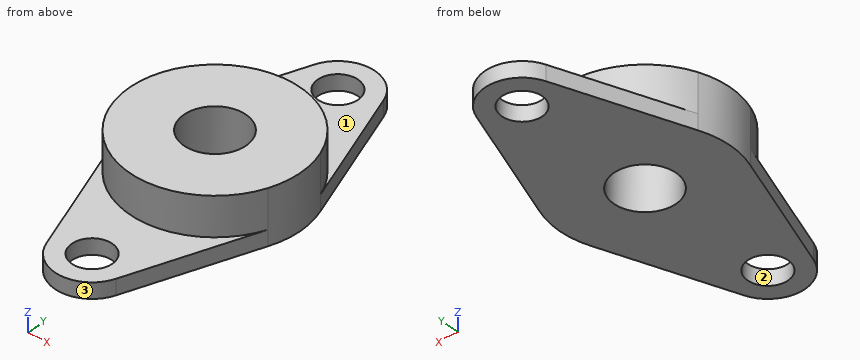
```python
from build123d import *

# Parameters (mm, degrees)
CROQUIS1_R              = 4
CROQUIS1_R_2            = 2.6
SALIENTE_EXTRUIR1_DEPTH = 7
CROQUIS2_R              = 2.6
CORTAR_EXTRUIR1_DEPTH   = 5


with BuildPart() as part:
    # Croquis1 → Saliente-Extruir1 (new body)
    with BuildSketch(Plane.XY):
        with BuildLine():
            Line((10.288824315, -3.891027397), (4.514634908, -19.880359362))
            ThreePointArc((4.514634908, -19.880359362), (0, -23.05), (-4.514634908, -19.880359362))
            Line((-4.514634908, -19.880359362), (-10.288824315, -3.891027397))
            ThreePointArc((-10.288824315, -3.891027397), (-11, 0), (-10.288824315, 3.891027397))
            Line((-10.288824315, 3.891027397), (-4.514634908, 19.880359362))
            ThreePointArc((-4.514634908, 19.880359362), (0, 23.05), (4.514634908, 19.880359362))
            Line((4.514634908, 19.880359362), (10.288824315, 3.891027397))
            ThreePointArc((10.288824315, 3.891027397), (11, 0), (10.288824315, -3.891027397))
        make_face()
        Circle(CROQUIS1_R, mode=Mode.SUBTRACT)
        with Locations((0, 18.25)):
            Circle(CROQUIS1_R_2, mode=Mode.SUBTRACT)
        with Locations((0, -18.25)):
            Circle(CROQUIS1_R_2, mode=Mode.SUBTRACT)
    extrude(amount=SALIENTE_EXTRUIR1_DEPTH)

    # Croquis2 → Cortar-Extruir1 (cut)
    with BuildSketch(Plane.XY.offset(7)):
        with BuildLine():
            Line((-4.514634908, 19.880359362), (-10.288824315, 3.891027397))
            ThreePointArc((-10.288824315, 3.891027397), (0, 11), (10.288824315, 3.891027397))
            Line((10.288824315, 3.891027397), (4.514634908, 19.880359362))
            ThreePointArc((4.514634908, 19.880359362), (0, 23.05), (-4.514634908, 19.880359362))
        make_face()
        with Locations((0, 18.25)):
            Circle(CROQUIS2_R, mode=Mode.SUBTRACT)
        with BuildLine():
            ThreePointArc((10.288824315, -3.891027397), (0, -11), (-10.288824315, -3.891027397))
            Line((-10.288824315, -3.891027397), (-4.514634908, -19.880359362))
            ThreePointArc((-4.514634908, -19.880359362), (0, -23.05), (4.514634908, -19.880359362))
            Line((4.514634908, -19.880359362), (10.288824315, -3.891027397))
        make_face()
        with Locations((0, -18.25)):
            Circle(CROQUIS2_R, mode=Mode.SUBTRACT)
    extrude(amount=-CORTAR_EXTRUIR1_DEPTH, mode=Mode.SUBTRACT)


solid = part.part
```
Design review of the part built by this model. Coordinates are the model's own, in mm. Face numbers are marked on the shaded views. Give positions to 0.01 mm unless a question says otherwise; leave off trailing zeros. Loops run counter-clockwise (first coordinate to the right, second up) from the corner with the lowest first, then second, coordinate; pieces in that order, holes last. Notation, with made-up numbers: (-6.5, 12.25) -> (21.5, 12.25) arc R31 cw to (21.5, 44.25) -> close; hole circle Ø5 at (-10.5, 39.5). An arc over 180 degrees is marked (long way). One line per item, written item: value.
Q1. Draft analysis for pull direction Y (two halves, no side actions). For the marked faces 1, 2 and 3, state which applies: pulls with the +Y half, pulls with the -Y half, needs draft (parallel to the pull), parting line crosses it, or undercut.
Numbers:
face 1: needs draft
face 2: undercut
face 3: pulls with the -Y half
Q2. We need section A-A on x = 0. Give the boundary of the cut face in (y, z).
Numbers:
outline: (-23.05, 0) -> (-20.85, 0) -> (-20.85, 2) -> (-23.05, 2) -> close; (-15.65, 0) -> (-4, 0) -> (-4, 7) -> (-11, 7) -> (-11, 2) -> (-15.65, 2) -> close; (4, 0) -> (15.65, 0) -> (15.65, 2) -> (11, 2) -> (11, 7) -> (4, 7) -> close; (20.85, 0) -> (23.05, 0) -> (23.05, 2) -> (20.85, 2) -> close
Q3. For pin 1 Ø6 at (x, y) = (7, -7.5) entering from -Z; pin 2 Ø8.5 at (x, y) = (0, -18.25) entering from +Z; pin 3 Ø3 at (y, z) = (-15.5, 3) entering from +X, all flat-tipped, find the tip position at first contact; note any pin that passes through.
Numbers:
pin 1: stops at z = 0
pin 2: stops at z = 2
pin 3: stops at x = 6.5
Q4. We need section B-B on z = 0.5. Give the boundary of the cut face in (x, y), and give its area (3 significant figures).
Numbers:
outline: (-10.29, -3.89) -> (-4.51, -19.88) arc R4.8 ccw to (4.51, -19.88) -> (10.29, -3.89) arc R11 ccw to (10.29, 3.89) -> (4.51, 19.88) arc R4.8 ccw to (-4.51, 19.88) -> (-10.29, 3.89) arc R11 ccw to start; hole circle Ø8 at (0, 0); hole circle Ø5.2 at (0, -18.25); hole circle Ø5.2 at (0, 18.25)
area: 590 mm^2
Q5. For L1, parallel to Y at x = 0, z = 1.2; L2, parallel to Y at x = 0, z = 5; L3, parallel to Z at x = -7.5, y = -9, list the stretches that pass through material, from the lowest coordinate up.
Numbers:
L1: y = -23.05 to -20.85, -15.65 to -4, 4 to 15.65, 20.85 to 23.05
L2: y = -11 to -4, 4 to 11
L3: z = 0 to 2
Q6. We need section D-D on z = 3.75. Give the boundary of the cut face in (x, y), and give its area (3 significant figures).
Numbers:
outline: circle Ø22 at (0, 0); hole circle Ø8 at (0, 0)
area: 330 mm^2
Q7. We need section C-C on y = 0. Give the boundary of the cut face in (x, z), and give its area (3 significant figures).
Numbers:
outline: (-11, 0) -> (-4, 0) -> (-4, 7) -> (-11, 7) -> close; (4, 0) -> (11, 0) -> (11, 7) -> (4, 7) -> close
area: 98.0 mm^2
